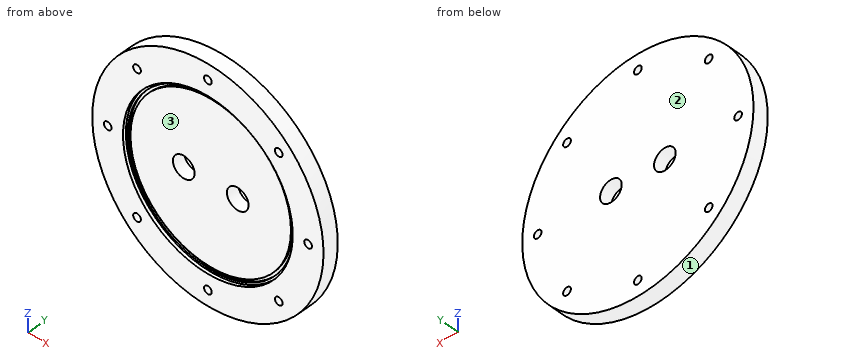
from build123d import *

# Parameters (mm, degrees)
SKETCH1_R                            = 95.25
BOSS_EXTRUDE1_DEPTH                  = 12.7
F_1_4_0_25_DIAMETER_HOLE1_D          = 6.35
CIRPATTERN1_COUNT                    = 8
SKETCH7_R                            = 69.9135
CUT_EXTRUDE3_DEPTH                   = 2.54
SKETCH2_R                            = 68.3133
SKETCH2_R_2                          = 66.1289
CUT_EXTRUDE1_DEPTH                   = 1.3208
F_45_64_0_70313_DIAMETER_HOLE1_D     = 17.859502
F_45_64_0_70313_DIAMETER_HOLE1_DEPTH = 25.4
F_45_64_0_70313_DIAMETER_HOLE1_TIP   = 5.365535714


with BuildPart() as part:
    # Sketch1 → Boss-Extrude1 (new body)
    with BuildSketch(Plane(origin=(0, 0, 0), x_dir=(1, 0, 0), z_dir=(0, 1, 0))):
        with Locations(Location((0, 0, 0), (0, 0, 270))):
            Circle(SKETCH1_R)
    extrude(amount=BOSS_EXTRUDE1_DEPTH)

    # 1/4 (0.25) Diameter Hole1 (through all)
    with Locations(Plane(origin=(0, 0, 0), x_dir=(-1, 0, 0), z_dir=(0, -1, 0))):
        with Locations((0, -82.55)):
            f_1_4_0_25_diameter_hole1 = Hole(F_1_4_0_25_DIAMETER_HOLE1_D / 2)

    # CirPattern1: 1/4 (0.25) Diameter Hole1 ×8 about axis
    cirpattern1_axis = Axis((0, 0, 0), (0, 1, 0))
    for i in range(1, CIRPATTERN1_COUNT):
        add(f_1_4_0_25_diameter_hole1.rotate(cirpattern1_axis, i * 360 / CIRPATTERN1_COUNT), mode=Mode.SUBTRACT)

    # Sketch7 → Cut-Extrude3 (cut)
    with BuildSketch(Plane(origin=(0, 0, 0), x_dir=(-1, 0, 0), z_dir=(0, -1, 0))):
        with Locations(Location((0, 0, 0), (0, 0, 90))):
            Circle(SKETCH7_R)
    extrude(amount=-CUT_EXTRUDE3_DEPTH, mode=Mode.SUBTRACT)

    # Sketch2 → Cut-Extrude1 (cut)
    with BuildSketch(Plane.XZ.offset(-2.54)):
        with Locations(Location((0, 0, 0), (0, 0, 270))):
            Circle(SKETCH2_R)
        with Locations(Location((0, 0, 0), (0, 0, 270))):
            Circle(SKETCH2_R_2, mode=Mode.SUBTRACT)
    extrude(amount=-CUT_EXTRUDE1_DEPTH, mode=Mode.SUBTRACT)

    # 45/64 (0.70313) Diameter Hole1
    with Locations(Plane(origin=(0, 2.54, 0), x_dir=(-1, 0, 0), z_dir=(0, -1, 0))):
        with Locations((22.225, 0), (-22.225, 0)):
            Hole(F_45_64_0_70313_DIAMETER_HOLE1_D / 2, depth=F_45_64_0_70313_DIAMETER_HOLE1_DEPTH)
            with Locations((0, 0, -(F_45_64_0_70313_DIAMETER_HOLE1_DEPTH + F_45_64_0_70313_DIAMETER_HOLE1_TIP / 2))):  # 118° drill point
                Cone(0, F_45_64_0_70313_DIAMETER_HOLE1_D / 2, F_45_64_0_70313_DIAMETER_HOLE1_TIP, mode=Mode.SUBTRACT)


solid = part.part
Read the model definition and answer for the solid it produces. Units are mm, in the model's axes. Face numbers are marked on the shaded views. Round coordinates to 2 decimals unless told otherwise and drop trailing zeros. Write each loop counter-clockwise with the first axis right and the second up, starting at its lowest first coordinate (ties: lowest second). Pieces come first, ordered by that corner, then holes.
Q1. Flat-ended cylindrical pins translate along their axes: P1, Ø5, axis at x = -38, y = 2, coming from the +Z side; P2, Ø2, axis at x = 18, y = 10.5, coming from the +Z side; P3, Ø4, axis at x = 69.5, y = 9.5, coming from the -Z side. Find the tip coordinate at first contact, or state that the pin passes through.
Values:
P1: stops at z = 88.39
P2: stops at z = 93.72
P3: stops at z = -67.2
Q2. Find section D-D on z = 82.55. Determine the outline of the cut face in (x, y) (3 decimals), and give its area (3 significant figures).
Values:
outline: (-47.519, 0) - (-3.175, 0) - (-3.175, 12.7) - (-47.519, 12.7) - close; (3.175, 0) - (47.519, 0) - (47.519, 12.7) - (3.175, 12.7) - close
area: 1,130 mm2
Q3. Straight lines are drawn through the part: line 1 (Z direction, x = 2.5, y = 10); line 2 (Z direction, x = 52, y = 2.75); line 3 (Y direction, x = 48, z = 3). For each, find the intervals that lie inside material, in ascending order.
Values:
line 1: z = -95.22 to -84.51, -80.59 to 80.59, 84.51 to 95.22
line 2: z = -79.8 to -44.3, -40.85 to 40.85, 44.3 to 79.8
line 3: y = 2.54 to 12.7
Q4. Find section A-A on z = 0. State how many separate pieces and enclosed holes the cut face has, and give its area (3 significant figures).
Values:
separate pieces: 5
enclosed holes: 0
area: 1,530 mm2
Q5. Find section B-B on x = 82.55. Determine the outline of the cut face in (y, z) (3 decimals).
Values:
outline: (0, -47.519) - (12.7, -47.519) - (12.7, -3.175) - (0, -3.175) - close; (0, 3.175) - (12.7, 3.175) - (12.7, 47.519) - (0, 47.519) - close
Q6. The mould has two halves that part along Z. Classify the marked faces 1, 2 and 3: released by +Z, released by -Z, zero draft, split by the parting line, or undercut.
Values:
face 1: split by the parting line
face 2: zero draft
face 3: undercut
